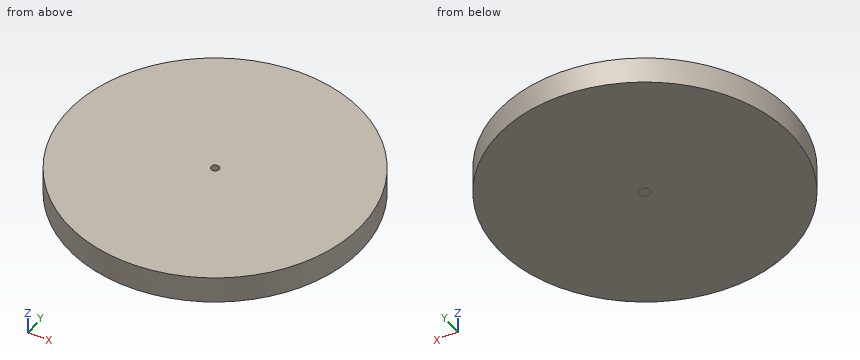
```python
from build123d import *

# Parameters (mm, degrees)
F0_R     = 27.5
F1_DEPTH = 5
F2_R     = 0.75
F3_DEPTH = 4.65
F4_R     = 0.25
F5_DEPTH = 2.35
F6_SIZE  = 0.25
F7_R     = 1
F8_DEPTH = 0.01


with BuildPart() as f1:
    # F0 (on Top) → F1 (new body)
    with BuildSketch(Plane.XY):
        Circle(F0_R)
    extrude(amount=F1_DEPTH)

    # F2 (on face) → F3 (cut)
    with BuildSketch(Plane.XY.offset(5)):
        Circle(F2_R)
    extrude(amount=-F3_DEPTH, mode=Mode.SUBTRACT)

    # F4 (on face) → F5 (join)
    with BuildSketch(Plane.XY.offset(0.35)):
        Circle(F4_R)
    extrude(amount=F5_DEPTH)

    # F6
    f6_edges = [f1.edges().sort_by_distance(p)[0] for p in [
        (-0.75, 0, 0.35),
    ]]
    chamfer(f6_edges, length=F6_SIZE)

    # F7 (on face) → F8 (join)
    with BuildSketch(Plane(origin=(0, 0, 0), x_dir=(1, 0, 0), z_dir=(0, 0, -1))):
        Circle(F7_R)
    extrude(amount=F8_DEPTH)


solid = f1.part
```
CAD build for the part. Positions are in the model's coordinates, mm. Round coordinates to 2 decimals unless told otherwise and drop trailing zeros. Order: outer loops, then holes, each group sorted by start corner. A loop starts at its lowest first (then second) coordinate and runs counter-clockwise, first axis right, second up. Notation, with made-up numbers: (-32.5, 68.25) - (-9.5, 68.25) arc R20 ccw to (-9.5, 98.25) - close; hole circle Ø7 at (49, 76.5). An arc over 180 degrees is marked (long way). Answer in a Markdown table with one row per item. Add a question column.
(1) Band-saw the part on C-C on x = 12. List the corners of the cut face in (y, z), and give its area (3 significant figures).
(2) Probe L1, parallel to Y at x = 0, z = 2.3; L2, parallel to Y at x = 0, z = 3.7; L3, parallel to Z at x = -18.5, y = 11. List the from-to ranges inside material, lowest first. Write a range as [from, to].
(3) Drop flat-ended pins along their axis: pin 1 Ø1.2 at (x, y) = (0, 0) entering from +Z; pin 2 Ø1 at (x, z) = (-11.5, 2.5) entering from -Y; pin 3 Ø2 at (x, y) = (13, -16.5) entering from -Z. Give the stop position or say it passes through.
(4) Band-saw the part on B-B on y = 10.5. List the corners of the cut face in (x, z).
(5) Band-saw the part on A-A on z = 1.6. List the corners of the cut face in (x, y).
Data:
| question | item | result |
|---|---|---|
| 1 | outline | (-24.74, 0) - (24.74, 0) - (24.74, 5) - (-24.74, 5) - close |
| 1 | area | 247 mm^2 |
| 2 | L1 | y = [-27.5, -0.75], [-0.25, 0.25], [0.75, 27.5] |
| 2 | L2 | y = [-27.5, -0.75], [0.75, 27.5] |
| 2 | L3 | z = [0, 5] |
| 3 | pin 1 | stops at z = 2.7 |
| 3 | pin 2 | stops at y = -25.2 |
| 3 | pin 3 | stops at z = 0 |
| 4 | outline | (-25.42, 0) - (25.42, 0) - (25.42, 5) - (-25.42, 5) - close |
| 5 | outline | circle Ø55 at (0, 0); circle Ø0.5 at (0, 0); hole circle Ø1.5 at (0, 0) |
